Part print with two shaded views. Sizes in mm from the minimum x, y, z corner. A direction names the side the tool comes from. Give positions to 0.01 mm unless a question says otherwise; leave off trailing zeros. Write each loop counter-clockwise with the first axis right and the second up, starting at its lowest first coordinate (ties: lowest second). Pieces come first, ordered by that corner, then holes.
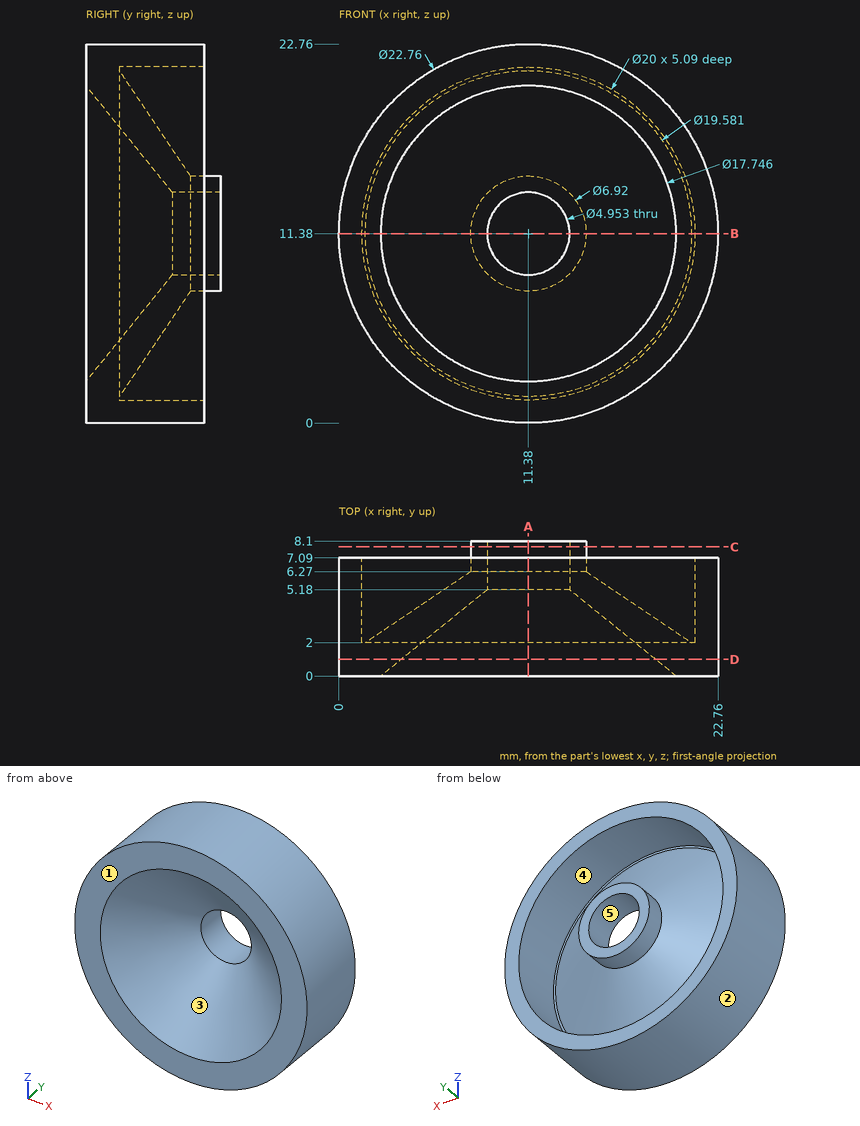
1) Flat gauge pins, fed straight in: P1, Ø1.5, axis at x = 18.5, y = 2, coming from the +Z side; P2, Ø3, axis at x = 5, y = 6, coming from the +Z side; P3, Ø4.5, axis at x = 11.38, z = 11.38, coming from the -Y side; P4, Ø3, axis at x = 16.5, y = 4.5, coming from the -Z side. Where does each tip first touch, or does it go through?
Check result:
P1: stops at z = 20.81
P2: stops at z = 21.66
P3: passes through
P4: stops at z = 0.59
2) Mould opens along X. For the marked faces 1, 2 and 3 say: +X half, -X half, draft (parallel to the pull), parting line (faces both ways), or undercut.
Check result:
face 1: draft
face 2: parting line
face 3: undercut
3) Saw through at A-A (x = 11.38). Write the cut outline in (y, z).
Check result:
outline: (0, 0) - (7.09, 0) - (7.09, 1.38) - (2, 1.38) - (2, 1.59) - (6.27, 7.92) - (8.1, 7.92) - (8.1, 8.9) - (5.18, 8.9) - (0, 2.51) - close; (0, 20.25) - (5.18, 13.86) - (8.1, 13.86) - (8.1, 14.84) - (6.27, 14.84) - (2, 21.17) - (2, 21.38) - (7.09, 21.38) - (7.09, 22.76) - (0, 22.76) - close
4) Saw through at B-B (z = 11.38). Write the cut outline in (x, y).
Check result:
outline: (0, 0) - (2.51, 0) - (8.9, 5.18) - (8.9, 8.1) - (7.92, 8.1) - (7.92, 6.27) - (1.59, 2) - (1.38, 2) - (1.38, 7.09) - (0, 7.09) - close; (13.86, 5.18) - (20.25, 0) - (22.76, 0) - (22.76, 7.09) - (21.38, 7.09) - (21.38, 2) - (21.17, 2) - (14.84, 6.27) - (14.84, 8.1) - (13.86, 8.1) - close
5) Saw through at C-C (y = 7.75). Write the cut outline in (x, z).
Check result:
outline: circle Ø6.92 at (11.38, 11.38); hole circle Ø4.95 at (11.38, 11.38)
6) Drill centre lines: L1, parallel to Z at x = 11.5, y = 7; L2, parallel to X at y = 6.8, z = 11.38; L3, parallel to X at y = 4, z = 11.38 (1 decimal). Where is each one in solid material? Low to high.
Check result:
L1: z = 0 to 1.38, 7.92 to 8.91, 13.85 to 14.84, 21.38 to 22.76
L2: x = 0 to 1.38, 7.92 to 8.9, 13.86 to 14.84, 21.38 to 22.76
L3: x = 0 to 1.4, 4.6 to 7.4, 15.3 to 18.2, 21.4 to 22.8
7) 3-axis set-ups, long thin cutter, end or side, ignore diameter. For the marked faces 4 and 5: which of +Z, -Z, +X, -X, +Y, -Y reach the whole face in a straight line?
Check result:
face 4: +Y
face 5: +Y, -Y
8) Saw through at D-D (y = 1). Write the cut outline in (x, z).
Check result:
outline: circle Ø22.76 at (11.38, 11.38); hole circle Ø15.28 at (11.38, 11.38)
